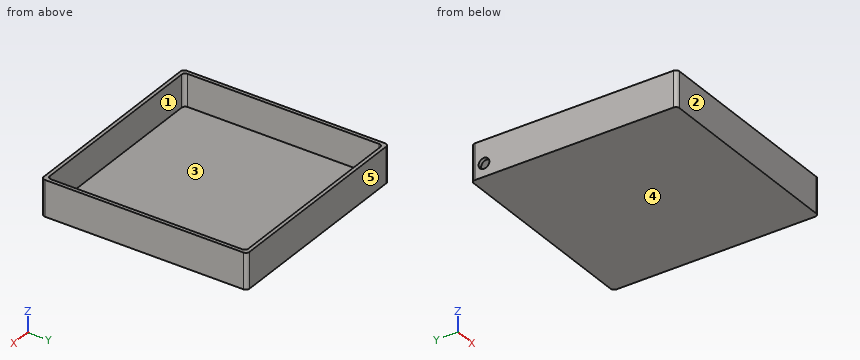
Autodesk Fusion 360 part; units mm, degrees
sketch "Esboço1" plane through (0, 0, 0) normal (0, 0, 1) x (1, 0, 0) in component "CASE"
  line L0 (-57.5, 57.5) -> (57.5, 57.5)
  line L1 (57.5, 57.5) -> (57.5, -57.5)
  line L2 (57.5, -57.5) -> (-57.5, -57.5)
  line L3 (-57.5, -57.5) -> (-57.5, 57.5)
  line L4 (-57.5, 57.5) -> (57.5, -57.5) construction
  line L5 (57.5, 57.5) -> (-57.5, -57.5) construction
  dimension "d5" = 115
  dimension "d6" = 115
sketch "Esboço2" plane through (0, 0, 0) normal (1, 0, 0) x (0, 1, 0) in component "CASE"
extrude "Extrusão1" add sketch "Esboço1" along normal blind 20 in component "CASE"
fillet "Arredondamento1" radius 4 4 edges at (57.5, -57.5, 10) (57.5, 57.5, 10) (-57.5, 57.5, 10) (-57.5, -57.5, 10) in component "CASE"
shell "Casca1" thickness 2 removed faces 1 at (-17.8333, -16.5, 20) in component "CASE"
delete_face "Excluir face1" 1 faces at (-55.3329, 57.0553, 6.6667) in component "CASE"
hole "Furo1" at (-57.5, 50.4054, 7.3062) direction (1, 0, 0) diameter 6 depth 4 tip angle 118 in component "CASE"
fillet "Arredondamento2" radius 2 1 edges at (-57.5, 57.5, 10) in component "CASE"
delete_face "Excluir face2" 1 faces at (-57.4955, -53.6903, 6.6667) in component "CASE"
fillet "Arredondamento3" radius 2 1 edges at (-57.5, -57.5, 10) in component "CASE"
delete_face "Excluir face3" 1 faces at (53.6903, -57.4955, 6.6667) in component "CASE"
fillet "Arredondamento4" radius 2 1 edges at (57.5, -57.5, 10) in component "CASE"
delete_face "Excluir face4" 1 faces at (55.3329, 57.0553, 6.6667) in component "CASE"
fillet "Arredondamento5" radius 2 1 edges at (57.5, 57.5, 10) in component "CASE"
component "CASE" placed x (1, 0, 0) y (0, 1, 0) z (0, 0, 1) at (0, 0, 0)
equation "COMPRIMENTO = 115 mm"
equation "ALTURA = 20 mm"
equation "SHELL = 2 mm"
equation "GAP = 0.2 mm"
equation "d5 = COMPRIMENTO"
equation "d6 = COMPRIMENTO"
equation "d7 = ALTURA"
equation "d11 = SHELL"
Geometry: final body of the model. Coordinates: model frame, mm. Face numbers are marked on the shaded views. A direction names the side the tool comes from. Round coordinates to 2 decimals unless told otherwise and drop trailing zeros. Order: outer loops, then holes, each group sorted by start corner. A loop starts at its lowest first (then second) coordinate and runs counter-clockwise, first axis right, second up. Notation, with made-up numbers: (86.25, -36) -> (98.25, -36) arc R26 cw to (98.25, -7) -> close; hole circle Ø10 at (-16.75, -7). An arc over 180 degrees is marked (long way). Write each question's results on one line, items separated by ' | '.
Q1. Section query D-D (z = 5.75). Output: boundary loops of the cut face in (x, y).
Response values:
outline: (-57.5, -55.5) arc R2 ccw to (-55.5, -57.5) -> (55.5, -57.5) arc R2 ccw to (57.5, -55.5) -> (57.5, 55.5) arc R2 ccw to (55.5, 57.5) -> (-55.5, 57.5) arc R2 ccw to (-57.5, 55.5) -> (-57.5, 52.97) -> (-55.5, 52.97) -> (-55.5, 53.5) arc R2 cw to (-53.5, 55.5) -> (53.5, 55.5) arc R2 cw to (55.5, 53.5) -> (55.5, -53.5) arc R2 cw to (53.5, -55.5) -> (-53.5, -55.5) arc R2 cw to (-55.5, -53.5) -> (-55.5, 47.84) -> (-57.5, 47.84) -> close
Q2. Pin query (flat end, axial travel): pin 1 Ø1 at (x, y) = (-39.5, 12) entering from +Z. Return the tip coordinate at first contact, or that it passes through.
Response values:
pin 1: z = 2
Q3. Pull-direction query (Y, two-part tool) for the marked faces 3, 4 and 5; classes: released by +Y, released by -Y, zero draft, split by the parting line, or undercut.
Response values:
face 3: undercut | face 4: zero draft | face 5: released by +Y
Q4. Ray query, line 1 along Y through (x, z) = (-27, 16.75); line 2 along Z through (x, y) = (-37.5, 48). Return the intervals inside material, ascending.
Response values:
line 1: -57.5 to -55.5, 55.5 to 57.5 | line 2: 0 to 2
Q5. Section query C-C (z = 14.25). Output: boundary loops of the cut face in (x, y).
Response values:
outline: (-57.5, -55.5) arc R2 ccw to (-55.5, -57.5) -> (55.5, -57.5) arc R2 ccw to (57.5, -55.5) -> (57.5, 55.5) arc R2 ccw to (55.5, 57.5) -> (-55.5, 57.5) arc R2 ccw to (-57.5, 55.5) -> close; hole (-55.5, -53.5) arc R2 ccw to (-53.5, -55.5) -> (53.5, -55.5) arc R2 ccw to (55.5, -53.5) -> (55.5, 53.5) arc R2 ccw to (53.5, 55.5) -> (-53.5, 55.5) arc R2 ccw to (-55.5, 53.5) -> close
Q6. Section query A-A (y = -33.5). Output: boundary loops of the cut face in (x, z).
Response values:
outline: (-57.5, 0) -> (57.5, 0) -> (57.5, 20) -> (55.5, 20) -> (55.5, 2) -> (-55.5, 2) -> (-55.5, 20) -> (-57.5, 20) -> close
Q7. Access query for the marked faces 1 and 2. Directions: +Z, -Z, +X, -X, +Y, -Y. A direction counts if a zero-diameter tool reaches every point of the face in a straight line with its end or side. Return the directions, or none.
Response values:
face 1: +Z | face 2: +Z, -Z, +X, -X, -Y
